The model under review builds one solid part; all positions refer to its coordinate system, in mm. A direction names the side the tool comes from. Coordinates: 2 decimals unless noted, no trailing zeros. Loops run counter-clockwise (first coordinate to the right, second up) from the corner with the lowest first, then second, coordinate; pieces in that order, holes last. Notation, with made-up numbers: M 46,11 L 76,11 A13 cw 76,32 Z; hole C -20,76 d2. An arc over 180 degrees is marked long. One line per item, written item: value.
```python
from build123d import *

# Parameters (mm, degrees)
BOSS_EXTRU_1_DEPTH       = 9.5
ESQUISSE3_R              = 2.5
ENL_V_MAT_EXTRU_40_DEPTH = 10
BOSS_EXTRU_2_DEPTH       = 2
CONG_1_R                 = 2
ESQUISSE5_R              = 6.5
BOSS_EXTRU_3_DEPTH       = 1.5
CONG_2_R                 = 0.75
ESQUISSE6_R              = 5.5
BOSS_EXTRU_4_DEPTH       = 0.5
ESQUISSE7_R              = 3
BOSS_EXTRU_5_DEPTH       = 3.5
ESQUISSE8_W              = 7
ESQUISSE8_H              = 4
BOSS_EXTRU_6_DEPTH       = 7


with BuildPart() as part:
    # Esquisse1 → Boss.-Extru.1 (new, symmetric)
    with BuildSketch(Plane(origin=(0, 0, 0), x_dir=(0, 0, -1), z_dir=(1, 0, 0))):
        Polygon((0, 0), (4, 0), (4, -7), (6, -7), (6, 0), (33, 0), (33, 40), (6, 40), (6, 47), (4, 47), (4, 40), (0, 40), align=None)
    extrude(amount=BOSS_EXTRU_1_DEPTH, both=True)

    # Esquisse3 → Enlèv. mat.-Extru.40 (cut)
    with BuildSketch(Plane.XY.offset(-4)):
        with Locations((5, 44.4)):
            Circle(ESQUISSE3_R)
        with Locations((-5, 44.4)):
            Circle(ESQUISSE3_R)
        with Locations((5, -4.4)):
            Circle(ESQUISSE3_R)
        with Locations((-5, -4.4)):
            Circle(ESQUISSE3_R)
    extrude(amount=-ENL_V_MAT_EXTRU_40_DEPTH, mode=Mode.SUBTRACT)

    # Esquisse4 → Boss.-Extru.2 (add)
    with BuildSketch(Plane.XY):
        with BuildLine():
            Line((-9.034932354, 5), (9.018945802, 5))
            Line((9.018945802, 5), (9.018945802, 29.110938176))
            ThreePointArc((9.018945802, 29.110938176), (-0.007993276, 40), (-9.034932354, 29.110938176))
            Line((-9.034932354, 29.110938176), (-9.034932354, 5))
        make_face()
    extrude(amount=BOSS_EXTRU_2_DEPTH)

    # Congé1
    cong_1_edges = [part.edges().sort_by_distance(p)[0] for p in [
        (-9.5, 20, -33),
        (0, 40, -33),
        (0, 0, -33),
        (9.5, 20, -33),
    ]]
    fillet(cong_1_edges, radius=CONG_1_R)

    # Esquisse5 → Boss.-Extru.3 (add)
    with BuildSketch(Plane.XY.offset(2)):
        with Locations(Location((0, 31.4090745, 0), (0, 0, 180))):
            Circle(ESQUISSE5_R)
    extrude(amount=BOSS_EXTRU_3_DEPTH)

    # Congé2
    cong_2_edges = [part.edges().sort_by_distance(p)[0] for p in [
        (6.5, 31.4090745, 3.5),
    ]]
    fillet(cong_2_edges, radius=CONG_2_R)

    # Esquisse6 → Boss.-Extru.4 (add)
    with BuildSketch(Plane.XY.offset(3.5)):
        with Locations((0, 31.4090745)):
            Circle(ESQUISSE6_R)
    extrude(amount=BOSS_EXTRU_4_DEPTH)

    # Esquisse7 → Boss.-Extru.5 (add)
    with BuildSketch(Plane.XY.offset(4)):
        with Locations((0, 31.4090745)):
            Circle(ESQUISSE7_R)
    extrude(amount=BOSS_EXTRU_5_DEPTH)

    # Esquisse8 → Boss.-Extru.6 (add)
    with BuildSketch(Plane(origin=(0, 40, 0), x_dir=(1, 0, 0), z_dir=(0, 1, 0))):
        with Locations((0, 30.314213562)):
            Rectangle(ESQUISSE8_W, ESQUISSE8_H)
    extrude(amount=BOSS_EXTRU_6_DEPTH)


solid = part.part
```
(1) To check wall thickness, follow L1, parallel to Y at x = 4.25, z = -3; L2, parallel to Z at x = 1, y = 43; L3, parallel to Z at x = 4.5, y = 9. State the ranges of each line that lie inside material, in increasing order. Write a range as [from, to].
Checks:
L1: [0, 40]
L2: [-32.31, -28.31], [-6, -4]
L3: [-33, 2]
(2) Insertion check: pin 1 Ø6.5 at (x, y) = (-5, -4.4) entering from -Z; pin 2 Ø2 at (y, z) = (45, -30.5) entering from -X; pin 3 Ø10 at (x, y) = (-7.5, 35.5) entering from +Z. Each pin has a flat end and moves straight along its axis. Give the tip position at first contact, or say it passes through.
Checks:
pin 1: z = -6
pin 2: x = -3.5
pin 3: z = 4
(3) Add section B-B on z = -29.5. State the section outline as (x, y) points.
Checks:
outline: M -9.5,0 L 9.5,0 L 9.5,40 L 3.5,40 L 3.5,47 L -3.5,47 L -3.5,40 L -9.5,40 Z
(4) Add section C-C on y = 44.4. State the section outline as (x, z) points.
Checks:
outline: M -9.5,-6 L -7.5,-6 L -7.5,-4 L -9.5,-4 Z; M -3.5,-32.31 L 3.5,-32.31 L 3.5,-28.31 L -3.5,-28.31 Z; M -2.5,-6 L 2.5,-6 L 2.5,-4 L -2.5,-4 Z; M 7.5,-6 L 9.5,-6 L 9.5,-4 L 7.5,-4 Z
(5) Tool access review of faces 5 (the face through (0, -4, -6)), 6 (the face through (0, 0, -2)), 7 (the face through (3.5, 43, -30)), 8 (the face through (0, 43, -32.314)): name each direction out of +Z, -Z, +X, -X, +Y, -Y from which nothing blocks a thin tool from reaching the whole face with its end or side.
Checks:
face 5: -Z, +X, -X, -Y
face 6: +Z, +X, -X, -Y
face 7: -Z, +X, +Y
face 8: -Z, +X, -X, +Y
(6) Add section A-A on y = -4.4. State the section outline as (x, z) points, then the cut area to 3 significant figures.
Checks:
outline: M -9.5,-6 L -7.5,-6 L -7.5,-4 L -9.5,-4 Z; M -2.5,-6 L 2.5,-6 L 2.5,-4 L -2.5,-4 Z; M 7.5,-6 L 9.5,-6 L 9.5,-4 L 7.5,-4 Z
area: 18.0 mm^2
(7) Draft analysis for pull direction Y (two halves, no side actions). For faces 1 (the face through (0, 47, -5)), 2 (the face through (6.34, 46.51, -4.99)), 3 (the face through (-3.66, 46.51, -4.99)), 4 (the face through (0, 5, 1)), state which applies: pulls with the +Y half, pulls with the -Y half, needs draft (parallel to the pull), parting line crosses it, or undercut.
Checks:
face 1: pulls with the +Y half
face 2: undercut
face 3: undercut
face 4: pulls with the -Y half
(8) Add section D-D on y = 22. State the section outline as (x, z) points.
Checks:
outline: M -9.5,-31 A2 ccw -7.5,-33 L 7.5,-33 A2 ccw 9.5,-31 L 9.5,0 L 9.02,0 L 9.02,2 L -9.03,2 L -9.03,0 L -9.5,0 Z
